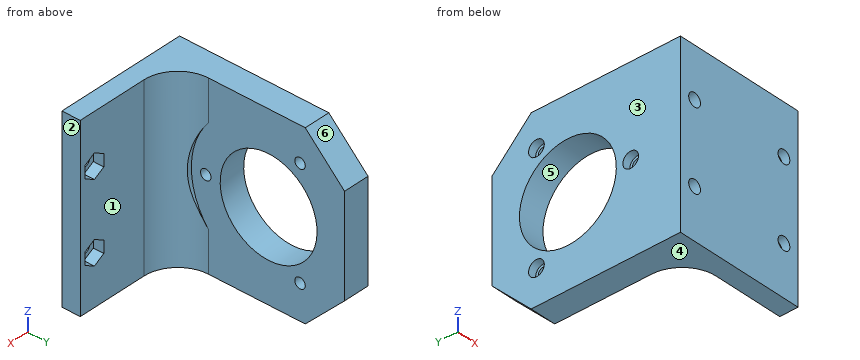
Autodesk Inventor part; units mm, degrees
ref_plane "YZ Plane" through (0, 0, 0) normal (1, 0, 0) x (0, 1, 0)
ref_plane "XZ Plane" through (0, 0, 0) normal (0, 1, 0) x (-1, 0, 0)
ref_plane "XY Plane" through (0, 0, 0) normal (0, 0, 1) x (1, 0, 0)
sketch "Skizze1" plane through (0, 0, 0) normal (0, 0, 1) x (1, 0, 0)
  line L0 (0, 0) -> (0, 72)
  line L1 (0, 72) -> (10, 72)
  line L2 (10, 72) -> (10, 7)
  line L3 (10, 7) -> (50, 7)
  line L4 (50, 7) -> (50, 0)
  line L5 (50, 0) -> (0, 0)
  dimension "d0" = 50
  dimension "d27" = 7
  dimension "d43" = 10
  dimension "d45" = 72
extrude "Extrusion1" add sketch "Skizze1" along normal mid plane 68
sketch "Skizze3" plane through (0, 0, 34) normal (0, -1, 0) x (1, 0, 0)
  line L0 (0, -68) -> (0, 0)
  line L1 (50, -68) -> (0, -68)
  point P0 (0, -34)
  point P1 (6, -49)
  point P2 (6, -19)
  dimension "d16" = 6
  dimension "d17" = 19
  dimension "d18" = 30
  dimension "d19" = 0
hole "Bohrung2" at (6, 0, -15) at (6, 0, 15) direction (0, 1, 0) diameter 5 depth 10
sketch "Skizze4" plane through (0, 0, 34) normal (0, -1, 0) x (1, 0, 0)
  circle A0 centre (6, -49) radius 2.5
  circle A1 centre (6, -19) radius 2.5
  point P0 (0, -34)
  point P1 (44, -49)
  point P2 (44, -19)
  dimension "d28" = 38
  dimension "d29" = 38
  dimension "d30" = 0
  dimension "d31" = 0
hole "Bohrung3" at (44, 0, -15) at (44, 0, 15) direction (0, 1, 0) diameter 5 end up to surface
sketch "Skizze5" plane through (10, 7, 34) normal (1, 0, 0) x (0, 0, -1)
  circle A0 centre (34, 36) radius 18.5
  line L0 (0, 0) -> (68, 0)
  point P0 (34, -7)
  dimension "d42" = 37
  dimension "d46" = 36
  dimension "d47" = 0
extrude "Extrusion2" cut sketch "Skizze5" against normal up to surface (10 mm away)
sketch "Skizze8" plane through (20, 7, 34) normal (0, 1, 0) x (1, 0, 0)
  circle A0 centre (24, 19) radius 2.5
  circle A1 centre (24, 49) radius 2.5
  line L0 (28, 21.3094) -> (28, 16.6906)
  line L1 (28, 16.6906) -> (24, 14.3812)
  line L2 (24, 14.3812) -> (20, 16.6906)
  line L3 (20, 16.6906) -> (20, 21.3094)
  line L4 (20, 21.3094) -> (24, 23.6188)
  line L5 (24, 23.6188) -> (28, 21.3094)
  line L6 (24, 44.3812) -> (20, 46.6906)
  line L7 (20, 46.6906) -> (20, 51.3094)
  line L8 (20, 51.3094) -> (24, 53.6188)
  line L9 (24, 53.6188) -> (28, 51.3094)
  line L10 (28, 51.3094) -> (28, 46.6906)
  line L11 (28, 46.6906) -> (24, 44.3812)
  line L12 (30, 0) -> (30, 68)
  point P0 (-20, 34)
  point P1 (24, 19)
  point P2 (24, 49)
  dimension "d54" = 8
  dimension "d55" = 8
extrude "Extrusion4" cut sketch "Skizze8" against normal blind 4
chamfer "Fase2" distance 15 angle 45 2 edges at (5, 72, -34) (5, 72, 34)
sketch "Skizze9" plane through (0, 0, -34) normal (-1, 0, 0) x (0, 0, 1)
  circle A0 centre (34, 43) radius 18.5
  circle A1 centre (34, 43) radius 18.5
  point P0 (34, 19)
  dimension "d84" = 0
  dimension "d85" = 24
hole "Bohrung4" at (0, 19, 0) direction (1, 0, 0) diameter 4 end up to surface counterbore diameter 6 counterbore depth 3
pattern_circular "Runde Anordnung1" count 3 over 360 about axis through (10, 43, 0) along (-1, 0, 0) of "Bohrung4"
fillet "Rundung1" radius 13 1 edges at (10, 7, 0)
sketch "Skizze11" plane through (10, 72, 19) normal (1, 0, 0) x (0, 0, -1)
  circle A0 centre (19, -29) radius 18.5
  circle A1 centre (19, -29) radius 18.5
  circle A2 centre (19, -29) radius 29.5
  point P0 (19, -72)
  dimension "d90" = 59
extrude "Extrusion5" cut sketch "Skizze11" along normal blind 10
equation "\"d55\" = d54"
properties part number "encoder_adapter" material "ABS Plastic"
The listing builds one solid part. Answer for the finished solid, in the listing's coordinates (mm). Face numbers are marked on the shaded views. A direction names the side the tool comes from. Coordinates: 2 decimals unless noted, no trailing zeros. Write each loop counter-clockwise with the first axis right and the second up, starting at its lowest first coordinate (ties: lowest second). Pieces come first, ordered by that corner, then holes. Notation, with made-up numbers: (15, 35) - (47, 35) arc R24 cw to (47, 68) - close; hole circle Ø8 at (84, 34.25). An arc over 180 degrees is marked (long way). Return JSON: item names as keys, results as strings.
1. Which of the six approach directions +Z, -Z, +X, -X, +Y, -Y give full straight-line access (tool end or side, diameter ignored) to the marked faces 1 and 2?
Final values:
{"face 1": "+Z, -Z, +X, +Y", "face 2": "+Z, -Z, +X, +Y, -Y"}
2. The part is cut by section C-C on x = 6. Determine the outline of the cut face in (y, z).
Final values:
{"outline": "(0, -34) - (57, -34) - (72, -19) - (72, 19) - (57, 34) - (0, 34) - (0, 17.5) - (10, 17.5) - (10, 12.5) - (0, 12.5) - (0, -12.5) - (10, -12.5) - (10, -17.5) - (0, -17.5) - close; hole circle Ø4 at (19, 0); hole circle Ø37 at (43, 0); hole circle Ø4 at (55, -20.78); hole circle Ø4 at (55, 20.78)"}
3. The part is cut by section D-D on z = -27.5. Determine the outline of the cut face in (x, y), then the cut area to 3 significant figures.
Final values:
{"outline": "(0, 0) - (50, 0) - (50, 7) - (23, 7) arc R13 cw to (10, 20) - (10, 63.5) - (0, 63.5) - close", "area": "951 mm^2"}
4. Consider line 1 along Z through (x, y) = (6, 5); line 2 along X through (y, z) = (3.75, -15); line 3 along X through (y, z) = (1.5, 15). Determine where each line is inside the solid, lowest interval first.
Final values:
{"line 1": "-34 to -17.5, -12.5 to 12.5, 17.5 to 34", "line 2": "0 to 3.5, 8.5 to 40, 48 to 50", "line 3": "0 to 3.5, 8.5 to 41.5, 46.5 to 50"}
5. The part is cut by section A-A on y = 43. Determine the outline of the cut face in (x, z), then the cut area to 3 significant figures.
Final values:
{"outline": "(0, -34) - (10, -34) - (10, -18.5) - (0, -18.5) - close; (0, 18.5) - (10, 18.5) - (10, 34) - (0, 34) - close", "area": "310 mm^2"}
6. The part is cut by section B-B on z = 0. Determine the outline of the cut face in (x, y).
Final values:
{"outline": "(0, 0) - (50, 0) - (50, 7) - (23, 7) arc R13 cw to (11.74, 13.5) - (10, 13.5) - (10, 17) - (3, 17) - (3, 16) - (0, 16) - close; (0, 22) - (3, 22) - (3, 21) - (10, 21) - (10, 24.5) - (0, 24.5) - close; (0, 61.5) - (10, 61.5) - (10, 72) - (0, 72) - close"}
7. Each of these flat-tipped pins is pushed along its axis until it touches: pin 1 Ø5 at (x, z) = (34.5, -12) entering from -Y; pin 2 Ø13.5 at (x, z) = (35.5, 17) entering from +Y; pin 3 Ø4 at (x, z) = (6, 15) entering from -Y; pin 4 Ø6 at (y, z) = (30, 23) entering from +X. Where does it stop, or does it pass through?
Final values:
{"pin 1": "y = 0", "pin 2": "y = 7", "pin 3": "y = 10", "pin 4": "x = 10"}
8. For a pull along Z with two mould halves and no side action, classify the marked faces 3, 4, 5 and 6 as +Z half, -Z half, draft (parallel to the pull), parting line (faces both ways), or undercut.
Final values:
{"face 3": "draft", "face 4": "-Z half", "face 5": "undercut", "face 6": "+Z half"}
